Check sheet for the modelled part. Datum: model origin and axes. Units: mm. Coordinates: 2 decimals unless noted, no trailing zeros. Loops run counter-clockwise (first coordinate to the right, second up) from the corner with the lowest first, then second, coordinate; pieces in that order, holes last. Notation, with made-up numbers: (20.5, 27) - (66.5, 27) arc R22 ccw to (66.5, 53) - close; hole circle Ø9 at (1, -35). An arc over 180 degrees is marked (long way). Use a Markdown table: item, result. Add a question column.
1) Sectioned sample at C-C, the plane z = 3.5. Enter the section's corners in (x, y), then the cut area to 3 significant figures.
2) Go/stop test with a flat-tipped pin: P1, Ø3, axis at x = 4, y = -4.5, coming from the +Z side. Record where the tip stops, or that it passes through.
3) Thickness scan on line 1 (Y direction, x = -0.25, z = 4.2); line 2 (X direction, y = -7.25, z = 2.5); line 3 (Y direction, x = 1, z = 3.4). Record the ranges inside material, lowest first.
4) Sectioned sample at A-A, the plane y = 0. Enter the section's corners in (x, z).
5) Draft check along Y on faces 1 (the cylindrical face through (4.38, -8.43, 2.46)), 2 (the flat face through (2.7, 9.3, 5)), 3 (the cylindrical face through (11.923, 3.755, 2.465)). Enter one of: pulls with the +Y half, pulls with the -Y half, needs draft (parallel to the pull), parting line crosses it, or undercut.
from build123d import *

# Parameters (mm, degrees)
CYLINDER001_R     = 9.5
CYLINDER001_DEPTH = 15
CYLINDER_R        = 12.5
CYLINDER_DEPTH    = 5


with BuildPart() as cilindro_interior:
    # Cylinder001 → Cylinder001 (new body)
    with BuildSketch(Plane.XY.offset(-4)):
        Circle(CYLINDER001_R)
    extrude(amount=CYLINDER001_DEPTH)


with BuildPart() as obj1:
    # Cylinder → Cylinder (new body)
    with BuildSketch(Plane.XY):
        Circle(CYLINDER_R)
    extrude(amount=CYLINDER_DEPTH)

    # Cut: cut Cilindro-interior
    add(cilindro_interior.part, mode=Mode.SUBTRACT)


solid = obj1.part
Solved:
| question | item | result |
|---|---|---|
| 1 | outline | circle Ø25 at (0, 0); hole circle Ø19 at (0, 0) |
| 1 | area | 207 mm2 |
| 2 | P1 | passes through |
| 3 | line 1 | y = -12.5 to -9.5, 9.5 to 12.5 |
| 3 | line 2 | x = -10.18 to -6.14, 6.14 to 10.18 |
| 3 | line 3 | y = -12.46 to -9.45, 9.45 to 12.46 |
| 4 | outline | (-12.5, 0) - (-9.5, 0) - (-9.5, 5) - (-12.5, 5) - close; (9.5, 0) - (12.5, 0) - (12.5, 5) - (9.5, 5) - close |
| 5 | face 1 | undercut |
| 5 | face 2 | needs draft |
| 5 | face 3 | parting line crosses it |
